Verification items for the finished model (mm, model axes). A direction names the side the tool comes from. Give positions to 0.01 mm unless a question says otherwise; leave off trailing zeros. Write each loop counter-clockwise with the first axis right and the second up, starting at its lowest first coordinate (ties: lowest second). Pieces come first, ordered by that corner, then holes. Notation, with made-up numbers: M 0,13.25 L 20,13.25 A23 cw 20,43.25 Z; hole C -20.75,38 d8. An arc over 180 degrees is marked long. Answer as a JSON object with one key per item and string values.
```python
from build123d import *

# Parameters (mm, degrees)
SALIENTE_EXTRUIR1_DEPTH = 6
CROQUIS7_R              = 40
SALIENTE_EXTRUIR5_DEPTH = 6
SALIENTE_EXTRUIR3_DEPTH = 6
CROQUIS6_R              = 1.75
SALIENTE_EXTRUIR4_DEPTH = 6
CROQUIS8_W              = 6
CROQUIS8_H              = 6
CORTAR_EXTRUIR1_DEPTH   = 25
CROQUIS9_W              = 322
CROQUIS9_H              = 247
CORTAR_EXTRUIR2_DEPTH   = 12
CROQUIS10_R             = 28.25
CORTAR_EXTRUIR3_DEPTH   = 6


with BuildPart() as part:
    # Croquis1 → Saliente-Extruir1 (new body)
    with BuildSketch(Plane(origin=(0, 0, 0), x_dir=(1, 0, 0), z_dir=(0, 1, 0))):
        with BuildLine():
            Line((-161, 103.5), (-38.791887254, 9.756509788))
            ThreePointArc((-38.791887254, 9.756509788), (-40, 0), (-38.791887254, -9.756509788))
            Line((-38.791887254, -9.756509788), (-161, -103.5))
            Line((-161, -103.5), (-161, -123.5))
            Line((-161, -123.5), (-141, -123.5))
            Line((-141, -123.5), (-22.823766962, -32.84928708))
            ThreePointArc((-22.823766962, -32.84928708), (0, -40), (22.823766962, -32.84928708))
            Line((22.823766962, -32.84928708), (141, -123.5))
            Line((141, -123.5), (161, -123.5))
            Line((161, -123.5), (161, -103.5))
            Line((161, -103.5), (38.791887254, -9.756509788))
            ThreePointArc((38.791887254, -9.756509788), (40, 0), (38.791887254, 9.756509788))
            Line((38.791887254, 9.756509788), (161, 103.5))
            Line((161, 103.5), (161, 123.5))
            Line((161, 123.5), (141, 123.5))
            Line((141, 123.5), (22.823766962, 32.84928708))
            ThreePointArc((22.823766962, 32.84928708), (0, 40), (-22.823766962, 32.84928708))
            Line((-22.823766962, 32.84928708), (-141, 123.5))
            Line((-141, 123.5), (-161, 123.5))
            Line((-161, 123.5), (-161, 103.5))
        make_face()
    extrude(amount=SALIENTE_EXTRUIR1_DEPTH)

    # Croquis7 → Saliente-Extruir5 (add)
    with BuildSketch(Plane(origin=(0, 0, 0), x_dir=(-1, 0, 0), z_dir=(0, -1, 0))):
        Circle(CROQUIS7_R)
    extrude(amount=SALIENTE_EXTRUIR5_DEPTH)

    # Croquis5 → Saliente-Extruir3 (add)
    with BuildSketch(Plane.XZ.offset(6)):
        with BuildLine():
            Line((18.896097481, -21), (-18.896097481, -21))
            ThreePointArc((-18.896097481, -21), (-28.25, 0), (-18.896097481, 21))
            Line((-18.896097481, 21), (-13.25, 21))
            Line((-13.25, 21), (-13.25, -11))
            Line((-13.25, -11), (13.25, -11))
            Line((13.25, -11), (13.25, 21))
            Line((13.25, 21), (18.896097481, 21))
            ThreePointArc((18.896097481, 21), (28.25, 0), (18.896097481, -21))
        make_face()
    extrude(amount=SALIENTE_EXTRUIR3_DEPTH)

    # Croquis6 → Saliente-Extruir4 (add)
    with BuildSketch(Plane.XZ.offset(12)):
        with BuildLine():
            Line((-18.896097481, 21), (-13.25, 21))
            Line((-13.25, 21), (-13.25, 3.5))
            ThreePointArc((-13.25, 3.5), (-13.103553391, 3.146446609), (-12.75, 3))
            Line((-12.75, 3), (12.75, 3))
            ThreePointArc((12.75, 3), (13.103553391, 3.146446609), (13.25, 3.5))
            Line((13.25, 3.5), (13.25, 21))
            Line((13.25, 21), (18.896097481, 21))
            ThreePointArc((18.896097481, 21), (28.25, 0), (18.896097481, -21))
            Line((18.896097481, -21), (-18.896097481, -21))
            ThreePointArc((-18.896097481, -21), (-28.25, 0), (-18.896097481, 21))
        make_face()
        with Locations((-8, -5.75)):
            Circle(CROQUIS6_R, mode=Mode.SUBTRACT)
        with Locations((8, -5.75)):
            Circle(CROQUIS6_R, mode=Mode.SUBTRACT)
    extrude(amount=SALIENTE_EXTRUIR4_DEPTH)

    # Croquis8 → Cortar-Extruir1 (cut, through all)
    with BuildSketch(Plane.XZ.offset(18)):
        with Locations((-20, 0)):
            Rectangle(CROQUIS8_W, CROQUIS8_H)
        with Locations((20, 0)):
            Rectangle(CROQUIS8_W, CROQUIS8_H)
    extrude(amount=-CORTAR_EXTRUIR1_DEPTH, mode=Mode.SUBTRACT)

    # Croquis9 → Cortar-Extruir2 (cut)
    with BuildSketch(Plane(origin=(0, 6, 0), x_dir=(1, 0, 0), z_dir=(0, 1, 0))):
        Rectangle(CROQUIS9_W, CROQUIS9_H)
    extrude(amount=-CORTAR_EXTRUIR2_DEPTH, mode=Mode.SUBTRACT)

    # Croquis10 → Cortar-Extruir3 (cut)
    with BuildSketch(Plane(origin=(0, -18, 0), x_dir=(1, 0, 0), z_dir=(0, 1, 0))):
        Circle(CROQUIS10_R)
    extrude(amount=CORTAR_EXTRUIR3_DEPTH, mode=Mode.SUBTRACT)


solid = part.part
```
1) Section check C-C on z = 12.5. Record the boundary of the cut face in (x, y).
Completed:
{"outline": "M -25.33,-12 L -13.25,-12 L -13.25,-6 L -25.33,-6 Z; M 13.25,-12 L 25.33,-12 L 25.33,-6 L 13.25,-6 Z"}
2) Access from +Z, -Z, +X, -X, +Y, -Y to the whole of each face (thin tool, end or side, straight path). Record for faces 4 (the face through (16, -9, 21)), 5 (the face through (-17, -9, 0)), 6 (the face through (13.25, -9, 5)).
Completed:
{"face 4": "+Z, +X, -X, +Y, -Y", "face 5": "+Y, -Y", "face 6": "+Z, +Y, -Y"}
3) Release check for a two-part mould opening along X. For faces 1 (the face through (0, -9, -21)), 2 (the face through (23, -9, 0)), 3 (the face through (-28.25, -8.96, -0.33)) record: pulls with the +X half, pulls with the -X half, needs draft (parallel to the pull), parting line crosses it, or undercut.
Completed:
{"face 1": "needs draft", "face 2": "undercut", "face 3": "pulls with the -X half"}
4) Thickness scan on L1, parallel to Z at x = -17.5, y = -11.3; L2, parallel to X at y = -9.25, z = -2.5; L3, parallel to Z at x = 6, y = -10.65. Record the ranges inside material, lowest first.
Completed:
{"L1": "z = -21 to -3, 3 to 21", "L2": "x = -28.14 to -23, -17 to -13.25, 13.25 to 17, 23 to 28.14", "L3": "z = -21 to -11"}
5) Section check D-D on z = 2. Record the boundary of the cut face in (x, y).
Completed:
{"outline": "M -28.18,-12 L -23,-12 L -23,-6 L -28.18,-6 Z; M -17,-12 L -13.25,-12 L -13.25,-6 L -17,-6 Z; M 13.25,-12 L 17,-12 L 17,-6 L 13.25,-6 Z; M 23,-12 L 28.18,-12 L 28.18,-6 L 23,-6 Z"}
6) Section check B-B on y = -8.55. Record the boundary of the cut face in (x, z).
Completed:
{"outline": "M -18.9,-21 L 18.9,-21 A28.25 ccw 18.9,21 L 13.25,21 L 13.25,-11 L -13.25,-11 L -13.25,21 L -18.9,21 A28.25 ccw Z; hole M -23,-3 L -17,-3 L -17,3 L -23,3 Z; hole M 17,-3 L 23,-3 L 23,3 L 17,3 Z"}
7) Go/stop test with flat-tipped pins: pin 1 (1.5 mm diameter, centred on y = -8.5, z = -8, fed in from +X); pin 2 (1.8 mm diameter, centred on y = -10, z = 5, fed in from +X); pin 3 (1.8 mm diameter, centred on y = -10, z = 2, fed in from -X); pin 4 (3 mm diameter, centred on x = -20, y = -8.5, fed in from -Z). Record where each tip stops, or that it passes through.
Completed:
{"pin 1": "stops at x = 27.3", "pin 2": "stops at x = 27.95", "pin 3": "stops at x = -28.23", "pin 4": "stops at z = -21"}
8) Section check A-A on x = 18. Record the boundary of the cut face in (y, z).
Completed:
{"outline": "M -12,-21 L -6,-21 L -6,-3 L -12,-3 Z; M -12,3 L -6,3 L -6,21 L -12,21 Z"}
